Read the model definition and answer for the solid it produces. Units are mm, in the model's axes. A direction names the side the tool comes from. Give positions to 0.01 mm unless a question says otherwise; leave off trailing zeros. Order: outer loops, then holes, each group sorted by start corner. A loop starts at its lowest first (then second) coordinate and runs counter-clockwise, first axis right, second up.
Item 1: A cutting plane is placed at B-B (x = 18). Write down the section's boundary in (y, z).
Item 2: The mould has two halves that part along Y. Classify faces 1 (the face through (25.636, -4.794, 3.477)), 2 (the face through (10, -10.795, 6)), 3 (the face through (-15.508, 5.008, 5.293)), 4 (the face through (-19.939, 0, 9)): +Y half, -Y half, draft (parallel to the pull), parting line (faces both ways), or undercut.
Item 3: A cutting plane is placed at A-A (y = -1.5). Write down the section's boundary in (x, z) (3 decimals).
Item 4: Find the intervals of material crossed by line 1 along X through (y, z) = (6.5, 11.5) (3 decimals); line 2 along Y through (x, z) = (13.5, 4.75); line 3 along Z through (x, y) = (25.5, -5.25), in increasing order.
Item 5: Given pin 1 Ø3 at (y, z) = (4, 10) entering from +X; pin 2 Ø3 at (x, z) = (11, 7) entering from +Y (3 decimals); pin 3 Ø2.5 at (x, y) = (-5.5, -1.5) entering from +Z; pin 4 Ø3.5 at (x, z) = (6.5, 2.5) entering from -Y, each flat-ended and moving along its own axis, determine where each tip first touches the part or whether it passes through.
Item 6: A cutting plane is placed at C-C (z = 4.5). State how many separate pieces and enclosed holes the cut face has, plus the area to 3 significant figures.
Item 7: Which of the six approach directions +Z, -Z, +X, -X, +Y, -Y give full straight-line access (tool end or side, diameter ignored) to faces 5 (the face through (-14, 4, 3.683)), 6 (the face through (-24, 0, 6.858)), 7 (the face through (-19, -10.795, 6)), 8 (the face through (-15, 9.271, 3)), 9 (the face through (5, -9.271, 3))?
Autodesk Inventor part; units mm, degrees
ref_plane "Work Plane1" through (19.939, -9.271, 0) normal (1, 0, 0) x (0, 0, -1)
ref_plane "YZ Plane" through (0, 0, 0) normal (1, 0, 0) x (0, 1, 0)
ref_plane "XZ Plane" through (0, 0, 0) normal (0, 1, 0) x (-1, 0, 0)
sketch "Sketch1" plane through (0, 0, 0) normal (0, 0, 1) x (1, 0, 0)
  line L0 (-27.559, 9.271) -> (27.559, 9.271)
  line L1 (27.559, 9.271) -> (27.559, -9.271)
  line L2 (27.559, -9.271) -> (-27.559, -9.271)
  line L3 (-27.559, -9.271) -> (-27.559, 9.271)
  line L4 (-27.559, 9.271) -> (27.559, -9.271) construction
  point P0 (0, 0)
  point P1 (0, 0)
  dimension "d0" = 55.118
  dimension "d1" = 18.542
extrude "Extrusion1" add sketch "Sketch1" along normal blind 6.858
sketch "Sketch2" plane through (0, 0, 6.858) normal (0, 0, 1) x (1, 0, 0)
  line L0 (27.559, -9.271) -> (-27.559, -9.271)
  circle A0 centre (-23.876, 4.064) radius 1.905
  circle A1 centre (-23.876, -4.064) radius 1.905
  circle A2 centre (23.876, 4.064) radius 1.905
  circle A3 centre (23.876, -4.064) radius 1.905
  line L1 (-23.876, 4.064) -> (-23.876, -4.064) construction
  line L2 (-23.876, -4.064) -> (23.876, -4.064) construction
  line L3 (23.876, -4.064) -> (23.876, 4.064) construction
  line L4 (23.876, 4.064) -> (-23.876, 4.064) construction
  line L5 (-23.876, 4.064) -> (23.876, -4.064) construction
  point P0 (0, 0)
  point P1 (0, 0)
  dimension "d4" = 3.81
  dimension "d5" = 4.318
  dimension "d6" = 43.942
extrude "Extrusion2" cut sketch "Sketch2" against normal up to surface (6.858 mm away)
ref_plane "Work Plane1" through (19.939, -9.271, 0) normal (1, 0, 0) x (0, 0, -1)
sketch "Sketch3" plane through (19.939, -9.271, 0) normal (1, 0, 0) x (0, 0, -1)
  line L0 (0, 20.066) -> (-11.4173, 20.066)
  line L1 (-13.0048, 18.4785) -> (-13.0048, 0.0635)
  line L2 (-11.4173, -1.524) -> (0, -1.524)
  line L3 (0, -1.524) -> (0, 0)
  line L4 (0, 0) -> (-6.858, 0)
  line L5 (-6.858, 0) -> (-6.858, 18.542)
  line L6 (-6.858, 18.542) -> (0, 18.542)
  line L7 (0, 18.542) -> (0, 20.066)
  line L8 (0, 18.542) -> (0, 0)
  line L9 (-6.858, 18.542) -> (-6.858, 0)
  arc A0 (-11.4173, 20.066) -> (-13.0048, 18.4785) centre (-11.4173, 18.4785) ccw
  arc A1 (-13.0048, 0.0635) -> (-11.4173, -1.524) centre (-11.4173, 0.0635) ccw
  point P0 (0, 9.271)
  dimension "d10" = 1.524
  dimension "d11" = 13.0048
  dimension "d12" = 1.5875
extrude "Extrusion3" add sketch "Sketch3" against normal blind 1.27 contours L7 L6 L5 L4 L3 L2 A1 L1 A0 L0
pattern_linear "Rectangular Pattern1" count 5 spacing 9.652 along (-1, 0, 0) of "Extrusion3"
sketch "Sketch4" plane through (0, 0, 6.858) normal (0, 0, 1) x (1, 0, 0)
  line L0 (-18.669, 9.2075) -> (-18.669, -9.2075)
  line L1 (-10.287, 9.2075) -> (-10.287, -9.2075)
  line L2 (-9.017, 9.2075) -> (-9.017, -9.2075)
  line L3 (-0.635, 9.2075) -> (-0.635, -9.2075)
  line L4 (0.635, 9.2075) -> (0.635, -9.2075)
  line L5 (9.017, 9.2075) -> (9.017, -9.2075)
  line L6 (10.287, 9.2075) -> (10.287, -9.2075)
  line L7 (18.669, 9.2075) -> (18.669, -9.2075)
  line L8 (19.939, 9.2075) -> (19.939, -9.2075)
  circle A0 centre (-14.478, 4.064) radius 1.397
  circle A1 centre (-14.478, -4.064) radius 1.397
  line L9 (-14.478, 4.064) -> (-14.478, -4.064) construction
  line L10 (-37.6243, 0) -> (37.6243, 0) construction
  circle A2 centre (-4.826, 4.064) radius 1.397
  circle A3 centre (-4.826, -4.064) radius 1.397
  circle A4 centre (4.826, 4.064) radius 1.397
  circle A5 centre (4.826, -4.064) radius 1.397
  circle A6 centre (14.478, 4.064) radius 1.397
  circle A7 centre (14.478, -4.064) radius 1.397
  point P0 (0, 0)
  point P1 (0, 0)
  point P2 (-14.478, 0)
  dimension "d18" = 2.794
  dimension "d19" = 5.334
  dimension "d21" = 4.191
  dimension "d28" = 9.652
extrude "Extrusion4" cut sketch "Sketch4" against normal blind 3.175
sketch "Sketch5" plane through (0, 0, 6.858) normal (0, 0, 1) x (1, 0, 0)
  circle A0 centre (-14.478, -4.064) radius 1.397
sketch "Sketch6" plane through (0, 0, 6.858) normal (0, 0, 1) x (1, 0, 0)
  circle A0 centre (-14.478, 4.064) radius 1.397
sketch "Sketch7" plane through (0, 0, 6.858) normal (0, 0, 1) x (1, 0, 0)
  circle A0 centre (-4.826, -4.064) radius 1.397
sketch "Sketch8" plane through (0, 0, 6.858) normal (0, 0, 1) x (1, 0, 0)
  circle A0 centre (-4.826, 4.064) radius 1.397
sketch "Sketch9" plane through (0, 0, 6.858) normal (0, 0, 1) x (1, 0, 0)
  circle A0 centre (4.826, 4.064) radius 1.397
sketch "Sketch10" plane through (0, 0, 6.858) normal (0, 0, 1) x (1, 0, 0)
  circle A0 centre (14.478, -4.064) radius 1.397
sketch "Sketch11" plane through (0, 0, 6.858) normal (0, 0, 1) x (1, 0, 0)
  circle A0 centre (23.876, 4.064) radius 1.905
sketch "Sketch12" plane through (0, 0, 6.858) normal (0, 0, 1) x (1, 0, 0)
  circle A0 centre (23.876, -4.064) radius 1.905
properties part number "Terminal Block"
Response values:
1. outline: (-9.27, 0) - (9.27, 0) - (9.27, 6.86) - (-9.27, 6.86) - close
2. face 1: undercut
2. face 2: -Y half
2. face 3: undercut
2. face 4: draft
3. outline: (-27.559, 0) - (27.559, 0) - (27.559, 6.858) - (19.939, 6.858) - (19.939, 13.005) - (18.669, 13.005) - (18.669, 6.858) - (10.287, 6.858) - (10.287, 13.005) - (9.017, 13.005) - (9.017, 6.858) - (0.635, 6.858) - (0.635, 13.005) - (-0.635, 13.005) - (-0.635, 6.858) - (-9.017, 6.858) - (-9.017, 13.005) - (-10.287, 13.005) - (-10.287, 6.858) - (-18.669, 6.858) - (-18.669, 13.005) - (-19.939, 13.005) - (-19.939, 6.858) - (-27.559, 6.858) - close
4. line 1: x = -19.939 to -18.669, -10.287 to -9.017, -0.635 to 0.635, 9.017 to 10.287, 18.669 to 19.939
4. line 2: y = -9.27 to -5.06, -3.07 to 3.07, 5.06 to 9.27
4. line 3: z = 0 to 6.86
5. pin 1: stops at x = 19.94
5. pin 2: stops at y = 10.795
5. pin 3: stops at z = 6.86
5. pin 4: stops at y = -9.27
6. separate pieces: 1
6. enclosed holes: 12
6. area: 947 mm2
7. face 5: +Z
7. face 6: +Z, -X, +Y, -Y
7. face 7: +Z, -Z, +X, -X, -Y
7. face 8: +Z, -Z, +Y
7. face 9: +Z, -Z, -Y
